Read the model definition and answer for the solid it produces. Units are mm, in the model's axes. A direction names the side the tool comes from. Coordinates: 2 decimals unless noted, no trailing zeros. Write each loop counter-clockwise with the first axis right and the second up, starting at its lowest first coordinate (ties: lowest second). Pieces come first, ordered by that corner, then holes.
(1) The part is cut by section B-B, the plane z = 20. State how many separate pieces and enclosed holes the cut face has, and give its area (3 significant figures).
(2) Straight lines are drawn through the part: line 1 along Y through (x, z) = (0, 16); line 2 along Y through (x, z) = (24, 6.75); line 3 along X through (y, z) = (-45, 24). For each, find the intervals that lie inside material, in ascending order.
(3) Which of the six approach directions +Z, -Z, +X, -X, +Y, -Y give full straight-line access (tool end or side, diameter ignored) to faces 4 (the cylindrical face through (-15.796, 70.274, 26.303)), 5 (the flat face through (17, 17, 3)), 6 (the flat face through (-8, -104, 2.5))?
(4) Determine the mould class of faces 1 (the flat face through (27, -2, 15)), 2 (the flat face through (20, 67, 22.5)), 3 (the flat face through (0, 57, 18)) for opening direction Y: pulls with the +Y half, pulls with the -Y half, needs draft (parallel to the pull), parting line crosses it, or undercut.
(5) The part is cut by section A-A, the plane y = -40.5. Determine the outline of the cut face in (x, z).
(6) Given pin 1 (6.5 mm diameter, centred on x = 17.68, y = 102.68, fed in from +Z); pin 2 (5 mm diameter, centred on x = -21, z = 17, fed in from +Y); pin 3 (3 mm diameter, centred on x = -11, z = 24, fed in from -Y); pin 4 (2.5 mm diameter, centred on x = -17.68, y = -67.32, fed in from -Z), each flat-ended and moving along its own axis, determine where each tip first touches the part or whether it passes through.
```python
from build123d import *

# Parameters (mm, degrees)
SKETCH_1_W                = 54
SKETCH_1_H                = 220
EXTRUDE_1_DEPTH           = 30
SKETCH_2_W                = 42.2
SKETCH_2_H                = 48
CUT_EXTRUDE_1_DEPTH       = 25
SKETCH_3_W                = 42.2
SKETCH_3_H                = 48
CUT_EXTRUDE_2_DEPTH       = 25
CUT_EXTRUDE_3_DEPTH       = 6
CUT_EXTRUDE_13_DEPTH      = 6
SKETCH_18_W               = 42.7
SKETCH_18_H               = 42.7
CUT_EXTRUDE_9_DEPTH       = 2.5
SKETCH_9_R                = 20.35
SKETCH_9_R_2              = 2.1
CUT_EXTRUDE_4_DEPTH       = 28.5
SKETCH_16_W               = 42.7
SKETCH_16_H               = 42.7
CUT_EXTRUDE_7_DEPTH       = 2.5
SKETCH_13_R               = 20.35
SKETCH_13_R_2             = 2.1
CUT_EXTRUDE_6_DEPTH       = 28.5
EXTRUDE_3_DEPTH           = 30
CUT_EXTRUDE_8_REACH       = 32
SKETCH_17_R               = 1.5
SKETCH_21_R               = 3.5
CUT_EXTRUDE_11_DEPTH      = 1
CUT_EXTRUDE_11_DEPTH_BACK = 7.5
EXTRUDE_4_DEPTH           = 30
SKETCH_29_R               = 3.5
CUT_EXTRUDE_15_DEPTH      = 7.5
CUT_EXTRUDE_16_REACH      = 32
SKETCH_30_R               = 1.5


with BuildPart() as part:
    # 草图1 → 凸台-拉伸1 (new body)
    with BuildSketch(Plane.XY):
        Rectangle(SKETCH_1_W, SKETCH_1_H)
    extrude(amount=EXTRUDE_1_DEPTH)

    # 草图2 → 切除-拉伸1 (cut)
    with BuildSketch(Plane.XY.offset(30)):
        with Locations((0, 33)):
            Rectangle(SKETCH_2_W, SKETCH_2_H)
    extrude(amount=-CUT_EXTRUDE_1_DEPTH, mode=Mode.SUBTRACT)

    # 草图3 → 切除-拉伸2 (cut)
    with BuildSketch(Plane(origin=(0, 0, 30), x_dir=(-1, 0, 0), z_dir=(0, 0, -1))):
        with Locations((0, -33)):
            Rectangle(SKETCH_3_W, SKETCH_3_H)
    extrude(amount=CUT_EXTRUDE_2_DEPTH, mode=Mode.SUBTRACT)

    # 草图4 → 切除-拉伸3 (cut, through all)
    with BuildSketch(Plane.XY.offset(5)):
        with BuildLine():
            Line((11, 31), (11, 35))
            ThreePointArc((11, 35), (0, 46), (-11, 35))
            Line((-11, 35), (-11, 31))
            ThreePointArc((-11, 31), (0, 20), (11, 31))
        make_face()
        with BuildLine():
            Line((-14, 46.5), (-14, 50.5))
            ThreePointArc((-14, 50.5), (-15.5, 52), (-17, 50.5))
            Line((-17, 50.5), (-17, 46.5))
            ThreePointArc((-17, 46.5), (-15.5, 45), (-14, 46.5))
        make_face()
        with BuildLine():
            ThreePointArc((17, 50.5), (15.5, 52), (14, 50.5))
            Line((14, 50.5), (14, 46.5))
            ThreePointArc((14, 46.5), (15.5, 45), (17, 46.5))
            Line((17, 46.5), (17, 50.5))
        make_face()
        with BuildLine():
            Line((14, 19.5), (14, 15.5))
            ThreePointArc((14, 15.5), (15.5, 14), (17, 15.5))
            Line((17, 15.5), (17, 19.5))
            ThreePointArc((17, 19.5), (15.5, 21), (14, 19.5))
        make_face()
        with BuildLine():
            ThreePointArc((-17, 15.5), (-15.5, 14), (-14, 15.5))
            Line((-14, 15.5), (-14, 19.5))
            ThreePointArc((-14, 19.5), (-15.5, 21), (-17, 19.5))
            Line((-17, 19.5), (-17, 15.5))
        make_face()
    extrude(amount=-CUT_EXTRUDE_3_DEPTH, mode=Mode.SUBTRACT)

    # 草图26 → 切除-拉伸13 (cut, through all)
    with BuildSketch(Plane.XY.offset(5)):
        with BuildLine():
            Line((11, -31), (11, -35))
            ThreePointArc((11, -35), (0, -46), (-11, -35))
            Line((-11, -35), (-11, -31))
            ThreePointArc((-11, -31), (0, -20), (11, -31))
        make_face()
        with BuildLine():
            Line((-13.95, -15.5), (-13.95, -19.5))
            ThreePointArc((-13.95, -19.5), (-15.5, -21.05), (-17.05, -19.5))
            Line((-17.05, -19.5), (-17.05, -15.5))
            ThreePointArc((-17.05, -15.5), (-15.5, -13.95), (-13.95, -15.5))
        make_face()
        with BuildLine():
            Line((-13.95, -50.5), (-13.95, -46.5))
            ThreePointArc((-13.95, -46.5), (-15.5, -44.95), (-17.05, -46.5))
            Line((-17.05, -46.5), (-17.05, -50.5))
            ThreePointArc((-17.05, -50.5), (-15.5, -52.05), (-13.95, -50.5))
        make_face()
        with BuildLine():
            Line((13.95, -50.5), (13.95, -46.5))
            ThreePointArc((13.95, -46.5), (15.5, -44.95), (17.05, -46.5))
            Line((17.05, -46.5), (17.05, -50.5))
            ThreePointArc((17.05, -50.5), (15.5, -52.05), (13.95, -50.5))
        make_face()
        with BuildLine():
            Line((13.95, -15.5), (13.95, -19.5))
            ThreePointArc((13.95, -19.5), (15.5, -21.05), (17.05, -19.5))
            Line((17.05, -19.5), (17.05, -15.5))
            ThreePointArc((17.05, -15.5), (15.5, -13.95), (13.95, -15.5))
        make_face()
    extrude(amount=-CUT_EXTRUDE_13_DEPTH, mode=Mode.SUBTRACT)

    # 草图18 → 切除-拉伸9 (cut)
    with BuildSketch(Plane.XY):
        with Locations((0, -85)):
            Rectangle(SKETCH_18_W, SKETCH_18_H)
    extrude(amount=CUT_EXTRUDE_9_DEPTH, mode=Mode.SUBTRACT)

    # 草图9 → 切除-拉伸4 (cut, through all)
    with BuildSketch(Plane.XY.offset(2.5)):
        with Locations((0, -85)):
            Circle(SKETCH_9_R)
        with Locations((-17.67766953, -67.32233047)):
            Circle(SKETCH_9_R_2)
        with Locations((17.67766953, -67.32233047)):
            Circle(SKETCH_9_R_2)
        with Locations((17.67766953, -102.67766953)):
            Circle(SKETCH_9_R_2)
        with Locations((-17.67766953, -102.67766953)):
            Circle(SKETCH_9_R_2)
    extrude(amount=CUT_EXTRUDE_4_DEPTH, mode=Mode.SUBTRACT)

    # 草图16 → 切除-拉伸7 (cut)
    with BuildSketch(Plane.XY):
        with Locations((0, 85)):
            Rectangle(SKETCH_16_W, SKETCH_16_H)
    extrude(amount=CUT_EXTRUDE_7_DEPTH, mode=Mode.SUBTRACT)

    # 草图13 → 切除-拉伸6 (cut, through all)
    with BuildSketch(Plane(origin=(0, 0, 2.5), x_dir=(-1, 0, 0), z_dir=(0, 0, -1))):
        with Locations((0, 85)):
            Circle(SKETCH_13_R)
        with Locations((-17.67766953, 102.67766953)):
            Circle(SKETCH_13_R_2)
        with Locations((17.67766953, 102.67766953)):
            Circle(SKETCH_13_R_2)
        with Locations((17.67766953, 67.32233047)):
            Circle(SKETCH_13_R_2)
        with Locations((-17.67766953, 67.32233047)):
            Circle(SKETCH_13_R_2)
    extrude(amount=-CUT_EXTRUDE_6_DEPTH, mode=Mode.SUBTRACT)

    # 草图15 → 凸台-拉伸3 (add)
    with BuildSketch(Plane(origin=(0, 0, 0), x_dir=(-1, 0, 0), z_dir=(0, 0, -1))):
        with BuildLine():
            Line((-27, 110), (27, 110))
            ThreePointArc((27, 110), (0, 121.796738986), (-27, 110))
        make_face()
    extrude(amount=-EXTRUDE_3_DEPTH)

    # 草图17 → 切除-拉伸8 (cut, up to next)
    with BuildSketch(Plane(origin=(0, 0, 0), x_dir=(-1, 0, 0), z_dir=(0, 0, -1)), mode=Mode.PRIVATE) as cut_extrude_8_sk1:
        with Locations((-24, 100)):
            Circle(SKETCH_17_R)
    cut_extrude_8_tool1 = extrude(cut_extrude_8_sk1.sketch, amount=-CUT_EXTRUDE_8_REACH, mode=Mode.PRIVATE) & part.part
    add(cut_extrude_8_tool1.solids().sort_by_distance((24, 100, 0))[0], mode=Mode.SUBTRACT)
    # 草图17 → 切除-拉伸8 (cut, up to next)
    with BuildSketch(Plane(origin=(0, 0, 0), x_dir=(-1, 0, 0), z_dir=(0, 0, -1)), mode=Mode.PRIVATE) as cut_extrude_8_sk2:
        with Locations((24, 100)):
            Circle(SKETCH_17_R)
    cut_extrude_8_tool2 = extrude(cut_extrude_8_sk2.sketch, amount=-CUT_EXTRUDE_8_REACH, mode=Mode.PRIVATE) & part.part
    add(cut_extrude_8_tool2.solids().sort_by_distance((-24, 100, 0))[0], mode=Mode.SUBTRACT)
    # 草图17 → 切除-拉伸8 (cut, up to next)
    with BuildSketch(Plane(origin=(0, 0, 0), x_dir=(-1, 0, 0), z_dir=(0, 0, -1)), mode=Mode.PRIVATE) as cut_extrude_8_sk3:
        with Locations((24, 66)):
            Circle(SKETCH_17_R)
    cut_extrude_8_tool3 = extrude(cut_extrude_8_sk3.sketch, amount=-CUT_EXTRUDE_8_REACH, mode=Mode.PRIVATE) & part.part
    add(cut_extrude_8_tool3.solids().sort_by_distance((-24, 66, 0))[0], mode=Mode.SUBTRACT)
    # 草图17 → 切除-拉伸8 (cut, up to next)
    with BuildSketch(Plane(origin=(0, 0, 0), x_dir=(-1, 0, 0), z_dir=(0, 0, -1)), mode=Mode.PRIVATE) as cut_extrude_8_sk4:
        with Locations((-24, 66)):
            Circle(SKETCH_17_R)
    cut_extrude_8_tool4 = extrude(cut_extrude_8_sk4.sketch, amount=-CUT_EXTRUDE_8_REACH, mode=Mode.PRIVATE) & part.part
    add(cut_extrude_8_tool4.solids().sort_by_distance((24, 66, 0))[0], mode=Mode.SUBTRACT)

    # 草图21 → 切除-拉伸11 (cut, two sides)
    with BuildSketch(Plane.XY.offset(30)) as cut_extrude_11_sk:
        with Locations((-17.67766953, 102.67766953)):
            Circle(SKETCH_21_R)
        with Locations((17.67766953, 102.67766953)):
            Circle(SKETCH_21_R)
        with Locations((17.67766953, 67.32233047)):
            Circle(SKETCH_21_R)
        with Locations((-17.67766953, 67.32233047)):
            Circle(SKETCH_21_R)
    extrude(amount=CUT_EXTRUDE_11_DEPTH, mode=Mode.SUBTRACT)
    extrude(cut_extrude_11_sk.sketch, amount=-CUT_EXTRUDE_11_DEPTH_BACK, mode=Mode.SUBTRACT)

    # 草图28 → 凸台-拉伸4 (add)
    with BuildSketch(Plane.XY.offset(30)):
        with BuildLine():
            Line((-27, -110), (27, -110))
            ThreePointArc((27, -110), (0, -121.795200461), (-27, -110))
        make_face()
    extrude(amount=-EXTRUDE_4_DEPTH)

    # 草图29 → 切除-拉伸15 (cut)
    with BuildSketch(Plane.XY.offset(30)):
        with Locations((-17.67766953, -67.32233047)):
            Circle(SKETCH_29_R)
        with Locations((17.67766953, -67.32233047)):
            Circle(SKETCH_29_R)
        with Locations((17.67766953, -102.67766953)):
            Circle(SKETCH_29_R)
        with Locations((-17.67766953, -102.67766953)):
            Circle(SKETCH_29_R)
    extrude(amount=-CUT_EXTRUDE_15_DEPTH, mode=Mode.SUBTRACT)

    # 草图30 → 切除-拉伸16 (cut, up to next)
    with BuildSketch(Plane(origin=(0, 0, 0), x_dir=(-1, 0, 0), z_dir=(0, 0, -1)), mode=Mode.PRIVATE) as cut_extrude_16_sk1:
        with Locations((-24, -100)):
            Circle(SKETCH_30_R)
    cut_extrude_16_tool1 = extrude(cut_extrude_16_sk1.sketch, amount=-CUT_EXTRUDE_16_REACH, mode=Mode.PRIVATE) & part.part
    add(cut_extrude_16_tool1.solids().sort_by_distance((24, -100, 0))[0], mode=Mode.SUBTRACT)
    # 草图30 → 切除-拉伸16 (cut, up to next)
    with BuildSketch(Plane(origin=(0, 0, 0), x_dir=(-1, 0, 0), z_dir=(0, 0, -1)), mode=Mode.PRIVATE) as cut_extrude_16_sk2:
        with Locations((-24, -66)):
            Circle(SKETCH_30_R)
    cut_extrude_16_tool2 = extrude(cut_extrude_16_sk2.sketch, amount=-CUT_EXTRUDE_16_REACH, mode=Mode.PRIVATE) & part.part
    add(cut_extrude_16_tool2.solids().sort_by_distance((24, -66, 0))[0], mode=Mode.SUBTRACT)
    # 草图30 → 切除-拉伸16 (cut, up to next)
    with BuildSketch(Plane(origin=(0, 0, 0), x_dir=(-1, 0, 0), z_dir=(0, 0, -1)), mode=Mode.PRIVATE) as cut_extrude_16_sk3:
        with Locations((24, -66)):
            Circle(SKETCH_30_R)
    cut_extrude_16_tool3 = extrude(cut_extrude_16_sk3.sketch, amount=-CUT_EXTRUDE_16_REACH, mode=Mode.PRIVATE) & part.part
    add(cut_extrude_16_tool3.solids().sort_by_distance((-24, -66, 0))[0], mode=Mode.SUBTRACT)
    # 草图30 → 切除-拉伸16 (cut, up to next)
    with BuildSketch(Plane(origin=(0, 0, 0), x_dir=(-1, 0, 0), z_dir=(0, 0, -1)), mode=Mode.PRIVATE) as cut_extrude_16_sk4:
        with Locations((24, -100)):
            Circle(SKETCH_30_R)
    cut_extrude_16_tool4 = extrude(cut_extrude_16_sk4.sketch, amount=-CUT_EXTRUDE_16_REACH, mode=Mode.PRIVATE) & part.part
    add(cut_extrude_16_tool4.solids().sort_by_distance((-24, -100, 0))[0], mode=Mode.SUBTRACT)


solid = part.part
```
Computed:
1. separate pieces: 1
1. enclosed holes: 20
1. area: 5,940 mm2
2. line 1: y = -121.8 to -105.35, -64.65 to -57, -9 to 9, 57 to 64.65, 105.35 to 121.8
2. line 2: y = -112.89 to -101.5, -98.5 to -67.5, -64.5 to 64.5, 67.5 to 98.5, 101.5 to 112.89
2. line 3: x = -27 to -21.1, 21.1 to 27
3. face 4: +Z
3. face 5: +Z, -Z
3. face 6: -Z
4. face 1: needs draft
4. face 2: undercut
4. face 3: undercut
5. outline: (-27, 0) - (-9.53, 0) - (-9.53, 5) - (-21.1, 5) - (-21.1, 30) - (-27, 30) - close; (9.53, 0) - (27, 0) - (27, 30) - (21.1, 30) - (21.1, 5) - (9.53, 5) - close
6. pin 1: stops at z = 22.5
6. pin 2: stops at y = 116.81
6. pin 3: stops at y = -120.55
6. pin 4: passes through
